```python
from build123d import *

# Parameters (mm, degrees)
F0_W      = 60
F0_H      = 37
F1_DEPTH  = 4
F3_DEPTH  = 4
F6_DEPTH  = 60
F8_W      = 52
F8_H      = 5
F7_W      = 52
F7_H      = 4
F9_DEPTH  = 25
F10_W     = 60
F10_H     = 4
F11_DEPTH = 10
F12_W     = 11
F12_H     = 6
F13_DEPTH = 4
F15_DEPTH = 60
F17_DEPTH = 25


with BuildPart() as f1:
    # F0 (on Top) → F1 (new body)
    with BuildSketch(Plane.XY):
        Rectangle(F0_W, F0_H)
    extrude(amount=-F1_DEPTH)

    # F4: F3 across plane


with BuildPart() as f3:
    # F2 (on face) → F3 (new body)
    with BuildSketch(Plane.YZ.offset(30)):
        with BuildLine():
            add(Edge.make_bspline(
                [(-18.5, 0), (-12.3333333333, 6.2487446703), (0, 15.7512553297), (12.3333333333, 6.2487446703), (18.5, 0)],
                knots=[0, 0, 0, 0, 0.5, 1, 1, 1, 1], degree=3))
            Line((-18.5, 0), (18.5, 0))
        make_face()
    extrude(amount=-F3_DEPTH)


with BuildPart() as f1_1:
    add(f1.part)
    add(f3.part.mirror(Plane.YZ))


    add(f3.part)  # F6 merges F3
    # F5 (on face) → F6 (join, through all)
    with BuildSketch(Plane.YZ.offset(30)):
        with BuildLine():
            add(Edge.make_bspline(
                [(-4.5, 0), (-4.6072629509, 4.5), (0.1894585205, 7.5), (4.22834591, 4.5), (4.5, 0)],
                knots=[0, 0, 0, 0, 0.5, 1, 1, 1, 1], degree=3))
            Line((-4.5, 0), (4.5, 0))
        make_face()
    extrude(amount=-F6_DEPTH)

    # F8 (on face) + F7 (on face) → F9 (cut)
    with BuildSketch(Plane.XY):
        with Locations((0, 7)):
            Rectangle(F8_W, F8_H)
    with BuildSketch(Plane.XY):
        with Locations((0, -6.5)):
            Rectangle(F7_W, F7_H)
    extrude(amount=-F9_DEPTH, mode=Mode.SUBTRACT)

    # F10 (on face) → F11 (join)
    with BuildSketch(Plane(origin=(0, 0, -4), x_dir=(1, 0, 0), z_dir=(0, 0, -1))):
        with Locations((0, 16.5)):
            Rectangle(F10_W, F10_H)
    extrude(amount=F11_DEPTH)

    # F12 (on face) → F13 (join)
    with BuildSketch(Plane(origin=(0, 0, -14), x_dir=(1, 0, 0), z_dir=(0, 0, -1))):
        with Locations((29.5, 17.5)):
            Rectangle(F12_W, F12_H)
        with Locations((-29.5, 17.5)):
            Rectangle(F12_W, F12_H)
    extrude(amount=-F13_DEPTH)

    # F14 (on face) → F15 (join, through all)
    with BuildSketch(Plane.YZ.offset(30)):
        Polygon((18.5, 0), (18.5, -4), (51.5, -14), (51.5, -10), align=None)
    extrude(amount=-F15_DEPTH)

    # F16 (on face) → F17 (cut)
    with BuildSketch(Plane(origin=(0, 1.5559293524, 5.1345668629), x_dir=(1, 0, 0), z_dir=(0, 0.2900073953, 0.9570244044))):
        with BuildLine():
            ThreePointArc((-10.3471690042, 46.7001105844), (0, 52.1868307812), (10.3471690042, 46.7001105844))
            Line((10.3471690042, 46.7001105844), (30, 17.704951482))
            Line((30, 17.704951482), (30, 52.1868307812))
            Line((30, 52.1868307812), (30, 58.4787502885))
            Line((30, 58.4787502885), (-30, 58.4787502885))
            Line((-30, 58.4787502885), (-30, 52.1868307812))
            Line((-30, 52.1868307812), (-30, 17.704951482))
            Line((-30, 17.704951482), (-10.3471690042, 46.7001105844))
        make_face()
    extrude(amount=-F17_DEPTH, mode=Mode.SUBTRACT)


solid = f1_1.part
```
The listing builds one solid part. Answer for the finished solid, in the listing's coordinates (mm). A direction names the side the tool comes from. Give positions to 0.01 mm unless a question says otherwise; leave off trailing zeros. Order: outer loops, then holes, each group sorted by start corner. A loop starts at its lowest first (then second) coordinate and runs counter-clockwise, first axis right, second up. Notation, with made-up numbers: (1, -21.75) - (34, -21.75) arc R26 ccw to (34, -7.75) - close; hole circle Ø3 at (26.5, -6.5). An arc over 180 degrees is marked (long way). Use one line per item in the form item = value. Start each with the question number.
(1) A cutting plane is placed at C-C, the plane y = 30. Write down the section's boundary in (x, z), then the cut area to 3 significant figures.
(2) A cutting plane is placed at A-A, the plane z = -6.25. Write down the section's boundary in (x, y) (3 decimals).
(3) Flat-ended cylindrical pins translate along their axes: pin 1 Ø6 at (x, y) = (-14, -2) entering from +Z; pin 2 Ø7 at (x, y) = (-4, 13.5) entering from +Z; pin 3 Ø1.2 at (x, z) = (-4.5, -1.5) entering from -Y. Find the tip coordinate at first contact, or state that the pin passes through.
(4) For faces 1 (the flat face through (0, -13, 0)), 2 (the flat face through (-26, 3, 5)), 3 (the flat face through (0, 14, 0)), determine the directions among +Z, -Z, +X, -X, +Y, -Y from which every point of the face is accessible in a straight line to the end or side of a thin tool.
(5) Consider line 1 (X direction, y = 7.5, z = -1.75); line 2 (X direction, y = 4, z = -3.5); line 3 (Z direction, x = -2.5, y = -15.5). Determine where each line is inside the solid, lowest interval first. Write a range as from..to.
(6) The mould has two halves that part along Y. Classify faces 4 (the flat face through (-30, -20.5, -12)), 5 (the flat face through (31, -18, -10)), 6 (the flat face through (0, -14.5, -9)), 7 (the flat face through (-20.31, 31.72, -5.67)): released by +Y, released by -Y, zero draft, split by the parting line, or undercut.
(7) A cutting plane is placed at B-B, the plane x = 1. State how many separate pieces and enclosed holes the cut face has, then the cut area to 3 significant figures.
Ans:
q1.outline = (-21.86, -3.48) - (-21.07, -7.48) - (21.07, -7.48) - (21.86, -3.48) - close
q1.area = 172 mm^2
q2.outline = (-30, -18.5) - (30, -18.5) - (30, -14.5) - (-30, -14.5) - close; (-23.955, 25.925) - (23.955, 25.925) - (15.393, 39.125) - (-15.393, 39.125) - close
q3.pin_1 = 6
q3.pin_2 = 0
q3.pin_3 = -18.5
q4.face_1 = +Z, -Y
q4.face_2 = +Z
q4.face_3 = +Z, +Y
q5.line_1 = -30..-26, 26..30
q5.line_2 = -30..30
q5.line_3 = -14..0
q6.face_4 = released by -Y
q6.face_5 = zero draft
q6.face_6 = undercut
q6.face_7 = released by +Y
q7.separate_pieces = 3
q7.enclosed_holes = 0
q7.area = 325 mm^2
